from build123d import *

# Parameters (mm, degrees)
SKETCH1_W           = 904.24
SKETCH1_H           = 114.3
SKETCH1_R           = 43.18
SKETCH1_R_2         = 9.525
BOSS_EXTRUDE1_DEPTH = 5.08
CHAMFER1_SIZE       = 25.4


with BuildPart() as part:
    # Sketch1 → Boss-Extrude1 (new body)
    with BuildSketch(Plane.XY):
        with Locations((452.12, 57.15)):
            Rectangle(SKETCH1_W, SKETCH1_H)
        with Locations((50.8, 57.15)):
            Circle(SKETCH1_R, mode=Mode.SUBTRACT)
        with Locations((860.552, 57.15)):
            Circle(SKETCH1_R_2, mode=Mode.SUBTRACT)
        with BuildLine():
            Line((301.752, 69.85), (708.152, 69.85))
            ThreePointArc((708.152, 69.85), (720.852, 57.15), (708.152, 44.45))
            Line((708.152, 44.45), (301.752, 44.45))
            ThreePointArc((301.752, 44.45), (289.052, 57.15), (301.752, 69.85))
        make_face(mode=Mode.SUBTRACT)
    extrude(amount=BOSS_EXTRUDE1_DEPTH)

    # Chamfer1
    chamfer1_edges = [part.edges().sort_by_distance(p)[0] for p in [
        (0, 114.3, 2.54),
        (904.24, 114.3, 2.54),
        (904.24, 0, 2.54),
        (0, 0, 2.54),
    ]]
    chamfer(chamfer1_edges, length=CHAMFER1_SIZE)


solid = part.part
Verification items for the finished model (mm, model axes). Give positions to 0.01 mm unless a question says otherwise; leave off trailing zeros. Order: outer loops, then holes, each group sorted by start corner. A loop starts at its lowest first (then second) coordinate and runs counter-clockwise, first axis right, second up. Notation, with made-up numbers: M 6.5,76 L 11.5,76 A18 cw 11.5,103 Z; hole C 54.25,59 d11. An arc over 180 degrees is marked long. Use one line per item in the form item = value. Start each with the question number.
Q1. Section check A-A (y = 57.15). Enter the section's corners in (x, z), then the cut area to 3 significant figures.
Q2. Scan lines: line 1 along Y through (x, z) = (402, 0.9); line 2 along X through (y, z) = (65, 0.95); line 3 along X through (y, z) = (63.5, 4.5). Record each from-to range of solid material in increasing order. Write a range as [from, to].
Q3. Section check C-C (x = 50.8). Enter the section's corners in (y, z), then the cut area to 3 significant figures.
Q4. Section check D-D (x = 326). Enter the section's corners in (y, z).
Q5. Section check B-B (z = 3.7). Enter the section's corners in (x, y) (3 decimals).
Q6. Mould release check, pull along X, two halves, no side actions. Record for faces 1 (the cylindrical face through (869.35, 53.5, 2.5)), 2 (the flat face through (446, 71, 5.08)), 3 (the flat face through (12.9, 12.5, 2.5)): +X half, -X half, draft (parallel to the pull), parting line (faces both ways), or undercut.
Evaluation:
q1.outline = M 0,0 L 7.62,0 L 7.62,5.08 L 0,5.08 Z; M 93.98,0 L 289.05,0 L 289.05,5.08 L 93.98,5.08 Z; M 720.85,0 L 851.03,0 L 851.03,5.08 L 720.85,5.08 Z; M 870.08,0 L 904.24,0 L 904.24,5.08 L 870.08,5.08 Z
q1.area = 1,860 mm2
q2.line_1 = [0, 44.45], [69.85, 114.3]
q2.line_2 = [0, 8.34], [93.26, 291.77], [718.14, 855.16], [865.95, 904.24]
q2.line_3 = [0, 8.09], [93.51, 290.75], [719.15, 853.45], [867.65, 904.24]
q3.outline = M 0,0 L 13.97,0 L 13.97,5.08 L 0,5.08 Z; M 100.33,0 L 114.3,0 L 114.3,5.08 L 100.33,5.08 Z
q3.area = 142 mm2
q4.outline = M 0,0 L 44.45,0 L 44.45,5.08 L 0,5.08 Z; M 69.85,0 L 114.3,0 L 114.3,5.08 L 69.85,5.08 Z
q5.outline = M 0,25.4 L 25.4,0 L 878.84,0 L 904.24,25.4 L 904.24,88.9 L 878.84,114.3 L 25.4,114.3 L 0,88.9 Z; hole C 50.8,57.15 d86.36; hole M 301.752,44.45 L 708.152,44.45 A12.7 ccw 708.152,69.85 L 301.752,69.85 A12.7 ccw Z; hole C 860.552,57.15 d19.05
q6.face_1 = undercut
q6.face_2 = draft
q6.face_3 = -X half
